The model under review builds one solid part; all positions refer to its coordinate system, in mm. A direction names the side the tool comes from. Round coordinates to 2 decimals unless told otherwise and drop trailing zeros. Write each loop counter-clockwise with the first axis right and the second up, starting at its lowest first coordinate (ties: lowest second). Pieces come first, ordered by that corner, then holes. Notation, with made-up numbers: (26, -25.5) - (83, -25.5) arc R19 ccw to (83, -15.5) - close; hole circle Ø1 at (11.5, 5.25). An arc over 180 degrees is marked (long way). Use one line per item in the form item = value.
from build123d import *

# Parameters (mm, degrees)
F0_R     = 44.45
F1_DEPTH = 25.4
F2_R     = 63.5
F2_R_2   = 44.45
F3_DEPTH = 127
F4_W     = 254
F4_H     = 50.8
F5_DEPTH = 152.4
F7_DEPTH = 120.65
F8_R     = 44.45
F9_DEPTH = 152.401


with BuildPart() as f1:
    # F0 (on Front) → F1 (new body)
    with BuildSketch(Plane.XZ):
        with BuildLine():
            Line((0, 50.8), (0, 0))
            Line((0, 0), (254, 0))
            Line((254, 0), (254, 50.8))
            Line((254, 50.8), (186.2277468166, 226.0981223472))
            ThreePointArc((186.2277468166, 226.0981223472), (127, 266.7), (67.7722531834, 226.0981223472))
            Line((67.7722531834, 226.0981223472), (0, 50.8))
        make_face()
        with Locations((127, 203.2)):
            Circle(F0_R, mode=Mode.SUBTRACT)
    extrude(amount=F1_DEPTH)

    # F2 (on face) → F3 (join)
    with BuildSketch(Plane.XZ.offset(25.4)):
        with Locations((127, 203.2)):
            Circle(F2_R)
        with Locations((127, 203.2)):
            Circle(F2_R_2, mode=Mode.SUBTRACT)
    extrude(amount=F3_DEPTH)

    # F4 (on face) → F5 (join)
    with BuildSketch(Plane.XZ.offset(25.4)):
        with Locations((127, 25.4)):
            Rectangle(F4_W, F4_H)
    extrude(amount=F5_DEPTH)

    # F6 (on face) → F7 (join)
    with BuildSketch(Plane.XZ.offset(25.4)):
        with BuildLine():
            ThreePointArc((139.7, 140.9829605333), (127, 139.7), (114.3, 140.9829605333))
            Line((114.3, 140.9829605333), (114.3, 50.8))
            Line((114.3, 50.8), (139.7, 50.8))
            Line((139.7, 50.8), (139.7, 140.9829605333))
        make_face()
    extrude(amount=F7_DEPTH)

    # F8 (on face) → F9 (cut, through all)
    with BuildSketch(Plane.XZ.offset(152.4)):
        with Locations((127, 203.2)):
            Circle(F8_R)
    extrude(amount=-F9_DEPTH, mode=Mode.SUBTRACT)


solid = f1.part
(1) Insertion check: P1, Ø5, axis at x = 166, y = -131, coming from the +Z side; P2, Ø4, axis at y = -35, z = 235, coming from the +X side; P3, Ø3, axis at y = -27, z = 220, coming from the +X side. Each pin has a flat end and moves straight along its axis. Give the tip position at first contact, or say it passes through.
Geometry results:
P1 = 255.16
P2 = 183.07
P3 = 188.63
(2) Add section C-C on x = 179. Write out the cut boundary in (y, z), then the cut area to 3 significant figures.
Geometry results:
outline = (-177.8, 0) - (0, 0) - (0, 239.65) - (-152.4, 239.65) - (-152.4, 166.75) - (-25.4, 166.75) - (-25.4, 50.8) - (-177.8, 50.8) - close
area = 23,100 mm2
(3) Add section D-D on z = 97.5. Write out the cut boundary in (x, y).
Geometry results:
outline = (18.05, -25.4) - (114.3, -25.4) - (114.3, -146.05) - (139.7, -146.05) - (139.7, -25.4) - (235.95, -25.4) - (235.95, 0) - (18.05, 0) - close
(4) To check wall thickness, follow L1, parallel to Z at x = 93, y = -33; L2, parallel to Z at x = 160.5, y = -141.5; L3, parallel to X at y = -47, z = 203. State the ranges of each line that lie inside material, in increasing order.
Geometry results:
L1 = 0 to 50.8, 149.57 to 174.57, 231.83 to 256.83
L2 = 0 to 50.8, 149.26 to 173.98, 232.42 to 257.14
L3 = 63.5 to 82.55, 171.45 to 190.5
(5) Add section B-B on x = 127. Write out the cut boundary in (y, z), then the cut area to 3 significant figures.
Geometry results:
outline = (-177.8, 0) - (0, 0) - (0, 158.75) - (-152.4, 158.75) - (-152.4, 139.7) - (-146.05, 139.7) - (-146.05, 50.8) - (-177.8, 50.8) - close; (-152.4, 247.65) - (0, 247.65) - (0, 266.7) - (-152.4, 266.7) - close
area = 27,800 mm2
(6) The part is to be moulded in two halves that separate along X. For faces 1 (the flat face through (125, 0, 106)), 2 (the cylindrical face through (150.9, -75.13, 240.68)), 3 (the flat face through (220.59, -12.52, 137.22)), say which applies: +X half, -X half, draft (parallel to the pull), parting line (faces both ways), or undercut.
Geometry results:
face_1 = draft
face_2 = undercut
face_3 = +X half
(7) Add section A-A on z = 203.2. Write out the cut boundary in (x, y).
Geometry results:
outline = (58.92, -25.4) - (63.5, -25.4) - (63.5, -152.4) - (82.55, -152.4) - (82.55, 0) - (58.92, 0) - close; (171.45, -152.4) - (190.5, -152.4) - (190.5, -25.4) - (195.08, -25.4) - (195.08, 0) - (171.45, 0) - close
(8) Machinability: for faces 4 (the flat face through (114.3, -85, 97)), 5 (the cylindrical face through (118.73, -92.07, 266.16)), 6 (the flat face through (139.7, -85, 95)), 7 (the flat face through (125, -177.8, 26)), 8 (the flat face through (140, -152.4, 246)), which of the approach directions +Z, -Z, +X, -X, +Y, -Y give a long, thin tool a straight path to every point of the face, cutting with its end or side? Answer none if there is none.
Geometry results:
face_4 = -X, -Y
face_5 = -Y
face_6 = +X, -Y
face_7 = +Z, -Z, +X, -X, -Y
face_8 = +Z, +X, -X, -Y
